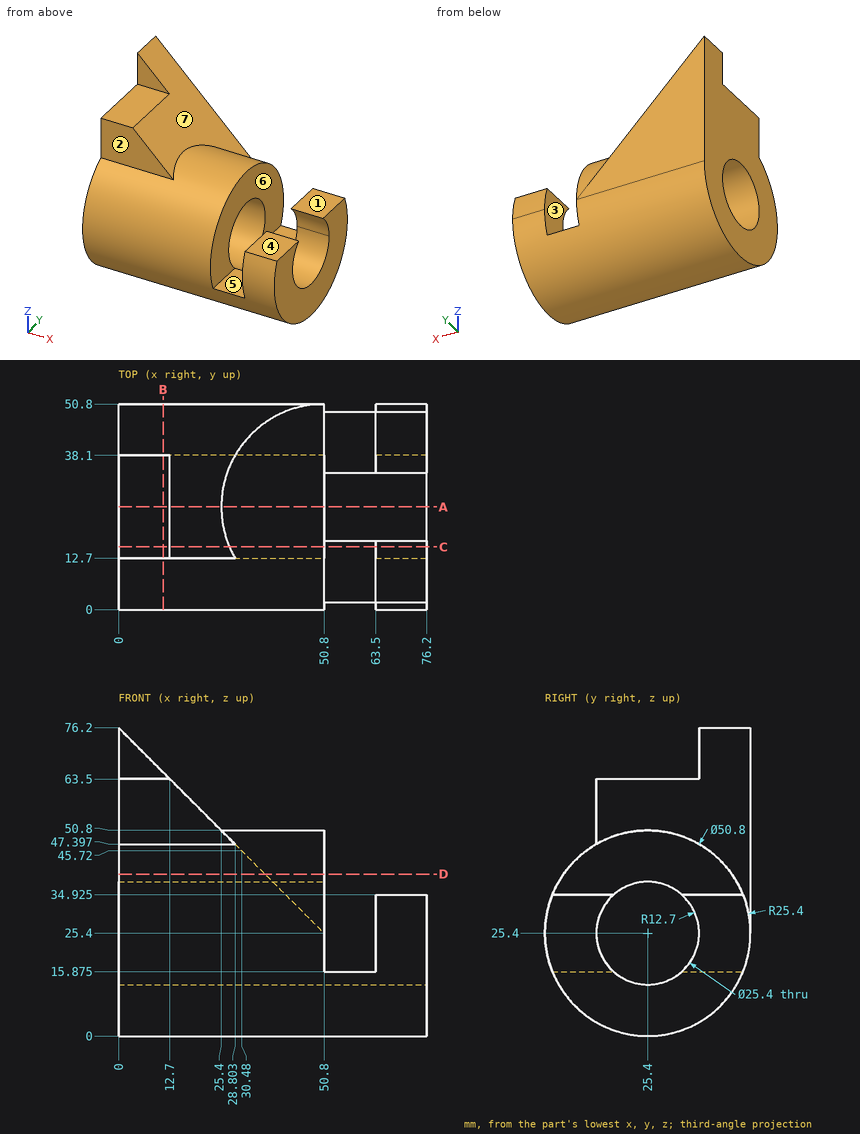
Part print with two shaded views. Sizes in mm from the minimum x, y, z corner. A direction names the side the tool comes from. Coordinates: 2 decimals unless noted, no trailing zeros. Write each loop counter-clockwise with the first axis right and the second up, starting at its lowest first coordinate (ties: lowest second). Pieces come first, ordered by that corner, then holes. Notation, with made-up numbers: (-23.5, -40) -> (25.5, -40) arc R15 ccw to (25.5, -11) -> close; hole circle Ø6 at (87, -36.75). An arc over 180 degrees is marked (long way). Return JSON: item names as keys, results as strings. Group by question number.
Q1. Cut at C-C, the plane y = 15.5. Give the cut face in (x, z) (3 decimals), then the cut area to 3 significant figures.
Q2. Which spindle directions (+Z, -Z, +X, -X, +Y, -Y) get a long thin tool onto all of the face, cutting with end or side? Do the marked faces 1, 2 and 3. Say none if no direction does.
Q3. Flat gauge pins, fed straight in: pin 1 (1.5 mm diameter, centred on x = 29.5, y = 31.5, fed in from -Z); pin 2 (14 mm diameter, centred on x = 59, y = 40.5, fed in from +Z) (3 decimals); pin 3 (5 mm diameter, centred on x = 20, y = 18.5, fed in from +Z). Where does each tip first touch, or does it go through?
Q4. Cut at A-A, the plane y = 25.4. Give the cut face in (x, z).
Q5. Pull direction X, two halves, no side cores. Call the marked faces 4, 5, 6 and 7: released by +X, released by -X, zero draft, split by the parting line, or undercut.
Q6. Cut at D-D, the plane z = 40. Give the cut face in (x, y).
Q7. Cut at B-B, the plane x = 11. Give the cut face in (y, z).
Q8. Drill centre lines: line 1 (X direction, y = 7, z = 16); line 2 (Z direction, x = 6, y = 25); line 3 (Y direction, x = 23, z = 26). Where is each one in solid material? Low to high.
Returned:
{
 "1": {"outline": "(0, 2.009) -> (76.2, 2.009) -> (76.2, 17.445) -> (63.5, 17.445) -> (63.5, 15.875) -> (50.8, 15.875) -> (50.8, 17.445) -> (0, 17.445) -> close; (0, 33.355) -> (50.8, 33.355) -> (50.8, 48.791) -> (27.409, 48.791) -> (12.7, 63.5) -> (0, 63.5) -> close; (63.5, 33.355) -> (76.2, 33.355) -> (76.2, 34.925) -> (63.5, 34.925) -> close", "area": "2,260 mm2"},
 "2": {"face 1": "+Z, +X, +Y, -Y", "face 2": "+Z, +X, -X, -Y", "face 3": "+Z, +Y, -Y"},
 "3": {"pin 1": "stops at z = 0.57", "pin 2": "stops at z = 34.925", "pin 3": "stops at z = 58.7"},
 "4": {"outline": "(0, 0) -> (76.2, 0) -> (76.2, 12.7) -> (0, 12.7) -> close; (0, 38.1) -> (50.8, 38.1) -> (50.8, 50.8) -> (25.4, 50.8) -> (12.7, 63.5) -> (0, 63.5) -> close"},
 "5": {"face 4": "zero draft", "face 5": "undercut", "face 6": "undercut", "face 7": "released by +X"},
 "6": {"outline": "(0, 4.62) -> (50.8, 4.62) -> (50.8, 46.18) -> (36.2, 46.18) -> (36.2, 50.8) -> (0, 50.8) -> close"},
 "7": {"outline": "(12.7, 47.4) arc R25.4 ccw (long way) to (50.8, 25.4) -> (50.8, 65.2) -> (38.1, 65.2) -> (38.1, 63.5) -> (12.7, 63.5) -> close; hole circle Ø25.4 at (25.4, 25.4)"},
 "8": {"line 1": "x = 0 to 50.8, 63.5 to 76.2", "line 2": "z = 0 to 12.71, 38.09 to 63.5", "line 3": "y = 0.01 to 12.71, 38.09 to 50.8"}
}
